For this review, take the finished solid that the model builds, in its own axes (mm). Round coordinates to 2 decimals unless told otherwise and drop trailing zeros. Write each loop counter-clockwise with the first axis right and the second up, starting at its lowest first coordinate (ties: lowest second). Pieces come first, ordered by that corner, then holes. Notation, with made-up numbers: (-5.75, 64) - (36.25, 64) arc R12 cw to (36.25, 87) - close; hole circle Ø6 at (32.25, -39). An arc over 180 degrees is marked (long way). Answer in a Markdown table with one row per item. Add a question column.
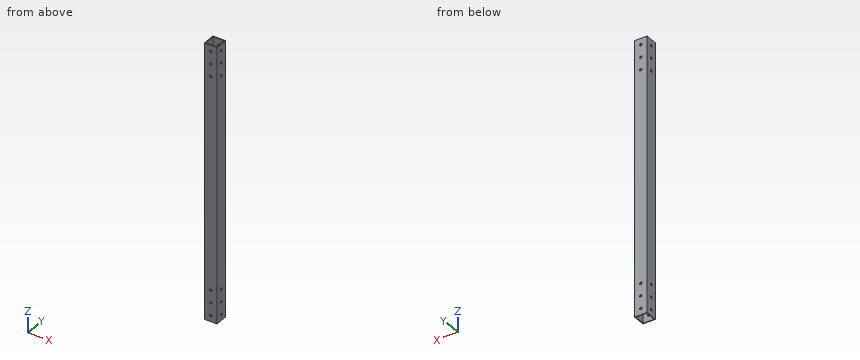
from build123d import *

# Parameters (mm, degrees)
SKETCH1_W           = 25.4
SKETCH1_H           = 25.4
BOSS_EXTRUDE1_DEPTH = 279.4
SHELL1_T            = -1.5875
SKETCH2_R           = 2.4892
CUT_EXTRUDE1_DEPTH  = 282.699627263
SKETCH3_R           = 2.4892
CUT_EXTRUDE2_DEPTH  = 282.699627263


with BuildPart() as part:
    # Sketch1 → Boss-Extrude1 (new, symmetric)
    with BuildSketch(Plane.XY):
        with Locations((12.7, 12.7)):
            Rectangle(SKETCH1_W, SKETCH1_H)
    extrude(amount=BOSS_EXTRUDE1_DEPTH, both=True)

    # Shell1
    shell1_openings = [part.faces().sort_by_distance(p)[0] for p in [
        (12.7, 12.7, 279.4),
        (12.7, 12.7, -279.4),
    ]]
    offset(amount=SHELL1_T, openings=shell1_openings, kind=Kind.INTERSECTION)

    # Sketch2 → Cut-Extrude1 (cut, through all)
    with BuildSketch(Plane(origin=(0, 25.4, 0), x_dir=(1, 0, 0), z_dir=(0, 1, 0))):
        with Locations(Location((12.7, -266.7, 0), (0, 0, 270))):
            Circle(SKETCH2_R)
        with Locations(Location((12.7, -241.3, 0), (0, 0, 270))):
            Circle(SKETCH2_R)
        with Locations(Location((12.7, -215.9, 0), (0, 0, 270))):
            Circle(SKETCH2_R)
    cut_extrude1 = extrude(amount=-CUT_EXTRUDE1_DEPTH, mode=Mode.SUBTRACT)

    # Sketch3 → Cut-Extrude2 (cut, through all)
    with BuildSketch(Plane.ZY):
        with Locations(Location((266.7, 12.7, 0), (0, 0, 270))):
            Circle(SKETCH3_R)
        with Locations(Location((241.3, 12.7, 0), (0, 0, 270))):
            Circle(SKETCH3_R)
        with Locations(Location((215.9, 12.7, 0), (0, 0, 270))):
            Circle(SKETCH3_R)
    cut_extrude2 = extrude(amount=-CUT_EXTRUDE2_DEPTH, mode=Mode.SUBTRACT)

    # Mirror1: Cut-Extrude1, Cut-Extrude2 across plane
    add(cut_extrude1.mirror(Plane.XY), mode=Mode.SUBTRACT)
    add(cut_extrude2.mirror(Plane.XY), mode=Mode.SUBTRACT)


solid = part.part
Q1. To check wall thickness, follow probe 1 along X at (y, z) = (3.25, -41); probe 2 along Y at (x, z) = (0.4, -241.3). State the ranges of each line that lie inside material, in increasing order.
Q2. Add section A-A on x = 19.25. State the section outline as (y, z) points.
Q3. Add section B-B on z = -86. State the section outline as (x, y) points.
Answer sheet:
| question | item | result |
|---|---|---|
| 1 | probe 1 | x = 0 to 1.59, 23.81 to 25.4 |
| 1 | probe 2 | y = 0 to 10.21, 15.19 to 25.4 |
| 2 | outline | (0, -279.4) - (1.59, -279.4) - (1.59, 279.4) - (0, 279.4) - close; (23.81, -279.4) - (25.4, -279.4) - (25.4, 279.4) - (23.81, 279.4) - close |
| 3 | outline | (0, 0) - (25.4, 0) - (25.4, 25.4) - (0, 25.4) - close; hole (1.59, 1.59) - (23.81, 1.59) - (23.81, 23.81) - (1.59, 23.81) - close |
